Autodesk Inventor part; units mm, degrees
ref_plane "YZ Plane" through (0, 0, 0) normal (1, 0, 0) x (0, 1, 0)
ref_plane "XZ Plane" through (0, 0, 0) normal (0, 1, 0) x (-1, 0, 0)
ref_plane "XY Plane" through (0, 0, 0) normal (0, 0, 1) x (1, 0, 0)
sketch "Sketch1" plane through (0, 0, 0) normal (0, 1, 0) x (-1, 0, 0)
  line L0 (0, 0) -> (-37.084, 0)
  line L1 (-37.084, 0) -> (-37.084, -43.942)
  line L2 (-37.084, -43.942) -> (0, -43.942)
  line L3 (0, -43.942) -> (0, 0)
  dimension "d0" = 43.942
  dimension "d1" = 37.084
extrude "Extrusion1" add sketch "Sketch1" along normal blind 17.78
sketch "Sketch2" plane through (0, 17.78, 0) normal (0, 1, 0) x (1, 0, 0)
  line L0 (0, 0) -> (37.084, 0)
  line L1 (37.084, 0) -> (11.684, 0)
  line L2 (11.684, 0) -> (11.684, 33.02)
  line L3 (11.684, 33.02) -> (37.084, 33.02)
  line L4 (37.084, 33.02) -> (37.084, 0)
  dimension "d4" = 33.02
  dimension "d5" = 25.4
extrude "Extrusion2" add sketch "Sketch2" along normal blind 12.7
sketch "Sketch3" plane through (0, 30.48, 0) normal (0, 1, 0) x (1, 0, 0)
  line L0 (37.084, 0) -> (37.084, 43.942)
  line L1 (16.256, 11.176) -> (37.084, 11.176)
  line L2 (37.084, 11.176) -> (37.084, 17.78)
  line L3 (37.084, 17.78) -> (16.256, 17.78)
  line L4 (16.256, 17.78) -> (16.256, 11.176)
  line L5 (11.684, 0) -> (37.084, 0)
  point P0 (0, 0)
  dimension "d8" = 17.78
  dimension "d9" = 6.604
  dimension "d10" = 20.828
extrude "Extrusion3" add sketch "Sketch3" along normal blind 25.4
sketch "Sketch4" plane through (0, 0, -43.942) normal (-1, 0, 0) x (0, 0, 1)
  line L0 (7.348, 15.289) -> (38.9211, 15.289) construction
  line L1 (38.9211, 15.289) -> (38.9211, 2.9854) construction
  line L2 (38.9211, 2.9854) -> (7.348, 2.9854) construction
  line L3 (7.348, 2.9854) -> (7.348, 15.289) construction
  point P0 (43.942, 0)
sketch "Sketch5" plane through (0, 0, 0) normal (0, -1, 0) x (1, 0, 0)
  circle A0 centre (18.542, -19.05) radius 19.812
  line L0 (0, 0) -> (37.084, 0)
  line L1 (37.084, -43.942) -> (0, -43.942) construction
  line L2 (18.542, -43.942) -> (18.542, 0) construction
  line L3 (11.684, 0) -> (37.084, 0) construction
  dimension "d13" = 39.624
  dimension "d14" = 19.05
extrude "Extrusion4" add sketch "Sketch5" along normal blind 17.78
properties part number "sierr olympic"
For this review, take the finished solid that the model builds, in its own axes (mm). A direction names the side the tool comes from. Round coordinates to 2 decimals unless told otherwise and drop trailing zeros. Order: outer loops, then holes, each group sorted by start corner. A loop starts at its lowest first (then second) coordinate and runs counter-clockwise, first axis right, second up. Notation, with made-up numbers: (31.25, 17) -> (66.25, 17) arc R20 cw to (66.25, 26) -> close; hole circle Ø5 at (-17, -9.5). An arc over 180 degrees is marked (long way). Use a Markdown table: item, result.
Item 1: For line 1 along X through (y, z) = (12, -37.5); line 2 along Z through (x, y) = (14, 30); line 3 along Y through (x, z) = (12.5, -18), list the stretches that pass through material, from the lowest coordinate up. Write a range as [from, to].
Resolved:
| item | result |
|---|---|
| line 1 | x = [0, 37.08] |
| line 2 | z = [-33.02, 0] |
| line 3 | y = [-17.78, 30.48] |
Item 2: Take a section at C-C (y = 33.5). State the section outline as (x, z) points, plus the area to 3 significant figures.
Resolved:
| item | result |
|---|---|
| outline | (16.26, -17.78) -> (37.08, -17.78) -> (37.08, -11.18) -> (16.26, -11.18) -> close |
| area | 138 mm² |
Item 3: For pin 1 (23 mm diameter, centred on x = 31, y = 41.5, fed in from +Z); pin 2 (8 mm diameter, centred on x = 15, z = -6, fed in from +Y); pin 3 (4 mm diameter, centred on y = 6.5, z = -27, fed in from +X); pin 4 (10 mm diameter, centred on x = 8.5, y = 40, fed in from +Z), all flat-tipped, find the tip position at first contact; note any pin that passes through.
Resolved:
| item | result |
|---|---|
| pin 1 | stops at z = 0 |
| pin 2 | stops at y = 30.48 |
| pin 3 | stops at x = 37.08 |
| pin 4 | passes through |
Item 4: Machinability: for faces 1 (the flat face through (11.684, 24, -16)), 2 (the flat face through (33, 0, -3)), 3 (the flat face through (4, 0, -3)), which of the approach directions +Z, -Z, +X, -X, +Y, -Y give a long, thin tool a straight path to every point of the face, cutting with its end or side? Answer none if there is none.
Resolved:
| item | result |
|---|---|
| face 1 | +Z, -Z, -X, +Y |
| face 2 | +Z, +X, -Y |
| face 3 | +Z, -X, -Y |
Item 5: Take a section at D-D (x = 22). State the section outline as (y, z) points.
Resolved:
| item | result |
|---|---|
| outline | (-17.78, -38.56) -> (0, -38.56) -> (0, -43.94) -> (17.78, -43.94) -> (17.78, -33.02) -> (30.48, -33.02) -> (30.48, -17.78) -> (55.88, -17.78) -> (55.88, -11.18) -> (30.48, -11.18) -> (30.48, 0) -> (0, 0) -> (0, 0.46) -> (-17.78, 0.46) -> close |
Item 6: Take a section at B-B (x = 7). State the section outline as (y, z) points, plus the area to 3 significant figures.
Resolved:
| item | result |
|---|---|
| outline | (-17.78, -35.15) -> (0, -35.15) -> (0, -43.94) -> (17.78, -43.94) -> (17.78, 0) -> (0, 0) -> (0, -2.95) -> (-17.78, -2.95) -> close |
| area | 1,350 mm² |
Item 7: Take a section at A-A (z = -19.05). State the section outline as (x, y) points, plus the area to 3 significant figures.
Resolved:
| item | result |
|---|---|
| outline | (-1.27, -17.78) -> (38.35, -17.78) -> (38.35, 0) -> (37.08, 0) -> (37.08, 30.48) -> (11.68, 30.48) -> (11.68, 17.78) -> (0, 17.78) -> (0, 0) -> (-1.27, 0) -> close |
| area | 1,690 mm² |
